Can you work these out from the model? Positions are in its coordinate system, mm. Face numbers are marked on the shaded views. A direction names the side the tool comes from. Give positions to 0.01 mm unless a question says otherwise; leave off trailing zeros. Answer as a JSON object with one key per item and string values.
```python
from build123d import *

# Parameters (mm, degrees)
SKICA1_R                 = 1.8
P_IDAT_VYSUNUT_M1_DEPTH  = 1.4
ODEBRAT_VYSUNUT_M1_DEPTH = 0.8
SKICA4_R                 = 1.05
P_IDAT_VYSUNUT_M2_DEPTH  = 6
ZKOSEN_1_SIZE            = 0.3
ZAOBLIT1_R               = 0.9


with BuildPart() as part:
    # Skica1 → Přidat vysunutím1 (new body)
    with BuildSketch(Plane.XY):
        Circle(SKICA1_R)
    extrude(amount=P_IDAT_VYSUNUT_M1_DEPTH)

    # Skica2 → Odebrat vysunutím1 (cut)
    with BuildSketch(Plane(origin=(0, 0, 0), x_dir=(-1, 0, 0), z_dir=(0, 0, -1))):
        Polygon((-0.443511417, 0.411741974), (-1.244198575, 0.411741974), (-1.244198575, -0.411741974), (-0.443511417, -0.411741974), (-0.443511417, -1.388921302), (0, -1.388921302), (0.443511417, -1.388921302), (0.443511417, -0.411741974), (1.244198575, -0.411741974), (1.244198575, 0.411741974), (0.443511417, 0.411741974), (0.443511417, 1.388921302), (0, 1.388921302), (-0.443511417, 1.388921302), align=None)
    extrude(amount=-ODEBRAT_VYSUNUT_M1_DEPTH, mode=Mode.SUBTRACT)

    # Skica4 → Přidat vysunutím2 (add)
    with BuildSketch(Plane.XY.offset(1.4)):
        Circle(SKICA4_R)
    extrude(amount=P_IDAT_VYSUNUT_M2_DEPTH)

    # Zkosení1
    zkosen_1_edges = [part.edges().sort_by_distance(p)[0] for p in [
        (-1.05, 0, 7.4),
    ]]
    chamfer(zkosen_1_edges, length=ZKOSEN_1_SIZE)

    # Zaoblit1
    # the kernel refuses this fillet: 0.9 mm, written as the material it takes off along each edge
    with BuildSketch(Plane(origin=(0, 0, 0), x_dir=(1, 0, 0), z_dir=(0, -1, 0))) as zaoblit1_piece_1:
        with BuildLine():
            CenterArc((1.8 - ZAOBLIT1_R, ZAOBLIT1_R), ZAOBLIT1_R, 270, 90)
            Line((1.8 - ZAOBLIT1_R, 0), (1.8, 0))
            Line((1.8, 0), (1.8, ZAOBLIT1_R))
        make_face()
    revolve(axis=Axis((0, 0, 0), (0, 0, 1)), mode=Mode.SUBTRACT)


solid = part.part
```
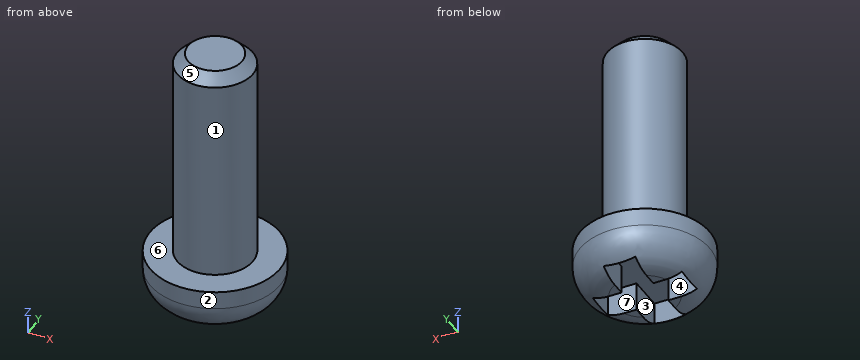
Q1. We'd pull the mould along Y, two halves only. Please class the marked faces 4, 5, 6 and 7: released by +Y, released by -Y, zero draft, split by the parting line, or undercut.
Recorded:
{"face 4": "undercut", "face 5": "split by the parting line", "face 6": "zero draft", "face 7": "undercut"}
Q2. Which directions (+Z, -Z, +X, -X, +Y, -Y) give clear straight access to the entire face, cutting with the end or side of a thin tool? Please do the marked faces 1, 2 and 3.
Recorded:
{"face 1": "+Z", "face 2": "+Z, -Z", "face 3": "-Z"}
Q3. I'm going to push flat-ended pins straight in: pin 1 Ø2 at (y, z) = (-1, 4.5) entering from -X; pin 2 Ø0.6 at (x, z) = (1, 0.5) entering from -Y; pin 3 Ø0.6 at (y, z) = (0, 0.5) entering from +X. Where does each tip first touch, or does it pass through?
Recorded:
{"pin 1": "stops at x = -1.05", "pin 2": "stops at y = -1.6", "pin 3": "stops at x = 1.79"}
Q4. I need wall thicknesses on L1, parallel to Z at x = 0.1, y = 1.1; L2, parallel to Y at x = 0.05, z = 5.25; L3, parallel to X at y = 0.35, z = 0.5. Which ranges of each line are inside material? Lowest first, please.
Recorded:
{"L1": "z = 0.8 to 1.4", "L2": "y = -1.05 to 1.05", "L3": "x = -1.67 to -1.24, 1.24 to 1.67"}
